```python
from build123d import *

# Parameters (mm, degrees)
F0_W     = 12.7
F0_H     = 12.7
F1_DEPTH = 6.35
F2_W     = 4.066467
F2_H     = 1.594322
F4_DEPTH = 4.699
F5_R     = 0.976004
F6_DEPTH = 25.4
F7_R     = 0.5


with BuildPart() as f1:
    # F0 (on Front) → F1 (new body)
    with BuildSketch(Plane.XZ):
        with Locations((1.14489, -0.153085)):
            Rectangle(F0_W, F0_H)
    extrude(amount=F1_DEPTH)

    # F2 (on face) → F4 (join)
    with BuildSketch(Plane.YZ.offset(7.49489)):
        with Locations((-3.161712, 2.55219)):
            Rectangle(F2_W, F2_H)
        with Locations((-3.161712, -2.55219)):
            Rectangle(F2_W, F2_H)
    extrude(amount=F4_DEPTH)

    # F5 (on face) → F6 (cut)
    with BuildSketch(Plane.XY.offset(3.349351)):
        with Locations((10.138705, -3.161712)):
            Circle(F5_R)
    extrude(amount=-F6_DEPTH, mode=Mode.SUBTRACT)

    # F7
    f7_edges = [f1.edges().sort_by_distance(p)[0] for p in [
        (1.14489, 0, 6.196915),
        (7.49489, 0, -0.153085),
        (7.49489, -3.175, 6.196915),
        (1.14489, -6.35, 6.196915),
        (-5.20511, -3.175, 6.196915),
        (7.49489, -6.35, -0.153085),
        (7.49489, -3.175, -6.503085),
        (-5.20511, 0, -0.153085),
        (1.14489, 0, -6.503085),
        (-5.20511, -6.35, -0.153085),
        (-5.20511, -3.175, -6.503085),
        (1.14489, -6.35, -6.503085),
    ]]
    fillet(f7_edges, radius=F7_R)


solid = f1.part
```
Could you check a few things on this model? Use its own coordinates, in mm. A direction names the side the tool comes from. Coordinates: 2 decimals unless noted, no trailing zeros. Loops run counter-clockwise (first coordinate to the right, second up) from the corner with the lowest first, then second, coordinate; pieces in that order, holes last. Notation, with made-up numbers: M 85,25.25 L 127,25.25 A16 cw 127,48.25 Z; hole C 1,-36 d4. An arc over 180 degrees is marked long. Put each result on its own line as item: value. Start each with the question number.
(1) Thinking about a two-plate mould opening in Z: for faces 6 (the face through (7.495, -3, 0)), 7 (the face through (10, -1.128, 3)), 8 (the face through (1, -3, -6.503)), which applies, pulls with the +Z half, pulls with the -Z half, needs draft (parallel to the pull), parting line crosses it, or undercut?
(2) I need wall thicknesses on line 1 (Z direction, x = 8.5, y = -3.5); line 2 (X direction, y = -4.75, z = -4.5); line 3 (Y direction, x = 8, z = 3). Which ranges of each line are inside material? Lowest first, please. Write a range as from..to.
(3) Suppose I cut it at C-C on z = -2.5. Please give me the cut outline in (x, y), then the cut area to 3 significant figures.
(4) Suppose I cut it at D-D on z = 5. Please give me the cut outline in (x, y).
(5) Will these pins go through, and if not, where does the flat tip stop? P1, Ø2, axis at x = 10.5, y = -4, coming from the +Z side; P2, Ø2, axis at x = 11, y = -2.5, coming from the -Z side; P3, Ø0.5, axis at x = 11, z = 3, coming from the +Y side; P4, Ø1.6, axis at x = 10.14, y = -3.16, coming from the -Z side.
(6) Suppose I cut it at A-A on y = -2. Please give me the cut outline in (x, z).
(7) For faces 1 (the face through (10, -1.128, -3)), 2 (the face through (9, -3, 3.349)), 3 (the face through (9, -3, -1.755)), 4 (the face through (9, -3, -3.349)), 5 (the face through (10, -5.195, 3)), which set-ups out of +Z, -Z, +X, -X, +Y, -Y let a thin tool reach every point of the face, with its end or its side?
(8) Suppose I cut it at B-B on x = 10.5. Please give me the cut outline in (y, z).
Solutions:
1. face 6: undercut
1. face 7: needs draft
1. face 8: pulls with the -Z half
2. line 1: z = -3.35..-1.76, 1.76..3.35
2. line 2: x = -5.21..7.49
2. line 3: y = -5.19..-1.13
3. outline: M -5.21,-5.85 A0.5 ccw -4.71,-6.35 L 6.99,-6.35 A0.5 ccw 7.49,-5.85 L 7.49,-5.19 L 12.19,-5.19 L 12.19,-1.13 L 7.49,-1.13 L 7.49,-0.5 A0.5 ccw 6.99,0 L -4.71,0 A0.5 ccw -5.21,-0.5 Z; hole C 10.14,-3.16 d1.95
3. area: 96.5 mm2
4. outline: M -5.21,-5.85 A0.5 ccw -4.71,-6.35 L 6.99,-6.35 A0.5 ccw 7.49,-5.85 L 7.49,-0.5 A0.5 ccw 6.99,0 L -4.71,0 A0.5 ccw -5.21,-0.5 Z
5. P1: stops at z = 3.35
5. P2: stops at z = -3.35
5. P3: stops at y = -1.13
5. P4: passes through
6. outline: M -5.21,-6 A0.5 ccw -4.71,-6.5 L 6.99,-6.5 A0.5 ccw 7.49,-6 L 7.49,-3.35 L 12.19,-3.35 L 12.19,-1.76 L 7.49,-1.76 L 7.49,1.76 L 12.19,1.76 L 12.19,3.35 L 7.49,3.35 L 7.49,5.7 A0.5 ccw 6.99,6.2 L -4.71,6.2 A0.5 ccw -5.21,5.7 Z
7. face 1: +Z, -Z, +X, +Y
7. face 2: +Z, +X, +Y, -Y
7. face 3: +X, +Y, -Y
7. face 4: -Z, +X, +Y, -Y
7. face 5: +Z, -Z, +X, -Y
8. outline: M -5.19,-3.35 L -4.07,-3.35 L -4.07,-1.76 L -5.19,-1.76 Z; M -5.19,1.76 L -4.07,1.76 L -4.07,3.35 L -5.19,3.35 Z; M -2.26,-3.35 L -1.13,-3.35 L -1.13,-1.76 L -2.26,-1.76 Z; M -2.26,1.76 L -1.13,1.76 L -1.13,3.35 L -2.26,3.35 Z
